from build123d import *

# Parameters (mm, degrees)
F0_R      = 4.75
F1_DEPTH  = 5
F2_R      = 7.5
F3_DEPTH  = 2
F4_R      = 3.825
F5_DEPTH  = 25
F6_R      = 0.25
F7_R      = 7.5
F7_R_2    = 6.65
F8_DEPTH  = 5
F9_R      = 5.0264335275
F9_R_2    = 3.825
F10_DEPTH = 1.2


with BuildPart() as f1:
    # F0 (on Top) → F1 (new body)
    with BuildSketch(Plane.XY):
        Circle(F0_R)
    extrude(amount=F1_DEPTH)

    # F2 (on face) → F3 (join)
    with BuildSketch(Plane.XY.offset(5)):
        Circle(F2_R)
    extrude(amount=F3_DEPTH)

    # F4 (on face) → F5 (cut)
    with BuildSketch(Plane.XY.offset(7)):
        Circle(F4_R)
    extrude(amount=-F5_DEPTH, mode=Mode.SUBTRACT)

    # F6
    f6_edges = [f1.edges().sort_by_distance(p)[0] for p in [
        (-7.5, 0, 7),
    ]]
    fillet(f6_edges, radius=F6_R)

    # F7 (on face) → F8 (join)
    with BuildSketch(Plane(origin=(0, 0, 5), x_dir=(1, 0, 0), z_dir=(0, 0, -1))):
        Circle(F7_R)
        Circle(F7_R_2, mode=Mode.SUBTRACT)
    extrude(amount=F8_DEPTH)

    # F9 (on face) → F10 (cut)
    with BuildSketch(Plane.XY.offset(7)):
        with Locations((0, -0.1200375191)):
            Circle(F9_R)
        Circle(F9_R_2, mode=Mode.SUBTRACT)
    extrude(amount=-F10_DEPTH, mode=Mode.SUBTRACT)


solid = f1.part
Verification items for the finished model (mm, model axes). A direction names the side the tool comes from. Give positions to 0.01 mm unless a question says otherwise; leave off trailing zeros. Write each loop counter-clockwise with the first axis right and the second up, starting at its lowest first coordinate (ties: lowest second). Pieces come first, ordered by that corner, then holes.
(1) Cross-section at A-A (x = 0). Enter the section's corners in (y, z) (3 decimals), plus the area to 3 significant figures.
(2) Cross-section at C-C (z = 6). Enter the section's corners in (x, y), plus the area to 3 significant figures.
(3) Mould release check, pull along X, two halves, no side actions. Record for faces 1 (the face through (-5, 2, 5)), 2 (the face through (-7.493, -0.33, 3.422)), 3 (the face through (2.192, -4.214, 2.465)), 4 (the face through (5, 2, 7)): +X half, -X half, draft (parallel to the pull), parting line (faces both ways), or undercut.
(4) Access from +Z, -Z, +X, -X, +Y, -Y to the whole of each face (thin tool, end or side, straight path). Record for faces 5 (the face through (-1, 7, 0)), 6 (the face through (2.7, 4.12, 6.41)), 7 (the face through (3.07, 5.9, 2.54)).
(5) Material ranges on line 1 (Y direction, x = 1.5, z = 3.75); line 2 (Y direction, x = 0, z = 3.25) (3 decimals); line 3 (X direction, y = 3.25, z = 0.5), recorded low to high.
(6) Cross-section at B-B (z = 4.75). Enter the section's corners in (x, y) (3 decimals).
(7) Gauge pin test, flat ends, axial feed: pin 1 (9 mm diameter, centred on x = 0, y = -0.12, fed in from +Z); pin 2 (3 mm diameter, centred on y = -3.5, z = 6, fed in from +X); pin 3 (5 mm diameter, centred on x = 6, y = -5.5, fed in from -Z); pin 4 (1 mm diameter, centred on y = -3, z = 3, fed in from -X). Record the tip position at first contact, or that the pin passes through.
Worked out:
1. outline: (-7.5, 0) - (-6.65, 0) - (-6.65, 5) - (-4.75, 5) - (-4.75, 0) - (-3.825, 0) - (-3.825, 5.8) - (-5.146, 5.8) - (-5.146, 7) - (-7.25, 7) arc R0.25 ccw to (-7.5, 6.75) - close; (3.825, 0) - (4.75, 0) - (4.75, 5) - (6.65, 5) - (6.65, 0) - (7.5, 0) - (7.5, 6.75) arc R0.25 ccw to (7.25, 7) - (4.906, 7) - (4.906, 5.8) - (3.825, 5.8) - close
1. area: 29.5 mm2
2. outline: circle Ø15 at (0, 0); hole circle Ø10.05 at (0, -0.12)
2. area: 97.3 mm2
3. face 1: undercut
3. face 2: parting line
3. face 3: undercut
3. face 4: draft
4. face 5: -Z, +X, -X, +Y, -Y
4. face 6: +Z
4. face 7: -Z
5. line 1: y = -7.35 to -6.48, -4.51 to -3.52, 3.52 to 4.51, 6.48 to 7.35
5. line 2: y = -7.5 to -6.65, -4.75 to -3.825, 3.825 to 4.75, 6.65 to 7.5
5. line 3: x = -6.76 to -5.8, -3.46 to -2.02, 2.02 to 3.46, 5.8 to 6.76
6. outline: circle Ø15 at (0, 0); circle Ø9.5 at (0, 0); hole circle Ø13.3 at (0, 0); hole circle Ø7.65 at (0, 0)
7. pin 1: stops at z = 5.8
7. pin 2: stops at x = 7.23
7. pin 3: stops at z = 0
7. pin 4: stops at x = -7.07
